```python
from build123d import *

# Parameters (mm, degrees)
SKETCH3_R           = 0.405
BOSS_EXTRUDE2_DEPTH = 70


with BuildPart() as part:
    # Sketch2 → Revolve1 (revolve)
    with BuildSketch(Plane.XY):
        Polygon((0, 0), (-9.85, 0), (-9.85, 4.95), (-3.328991597, 4.95), (-3.328991597, 5.45), (0, 5.45), align=None)
    revolve(axis=Axis((0, 5.45, 0), (0, -1, 0)))

    # Sketch3 → Boss-Extrude2 (add)
    with BuildSketch(Plane(origin=(0, 0, 0), x_dir=(0, 0, -1), z_dir=(1, 0, 0))):
        with Locations(Location((-0.41, 2.05, 0), (0, 0, 180))):
            Circle(SKETCH3_R)
        with Locations(Location((-1.23, 2.05, 0), (0, 0, 180))):
            Circle(SKETCH3_R)
        with Locations(Location((1.23, 2.05, 0), (0, 0, 180))):
            Circle(SKETCH3_R)
        with Locations(Location((0.41, 2.05, 0), (0, 0, 180))):
            Circle(SKETCH3_R)
    extrude(amount=BOSS_EXTRUDE2_DEPTH)


solid = part.part
```
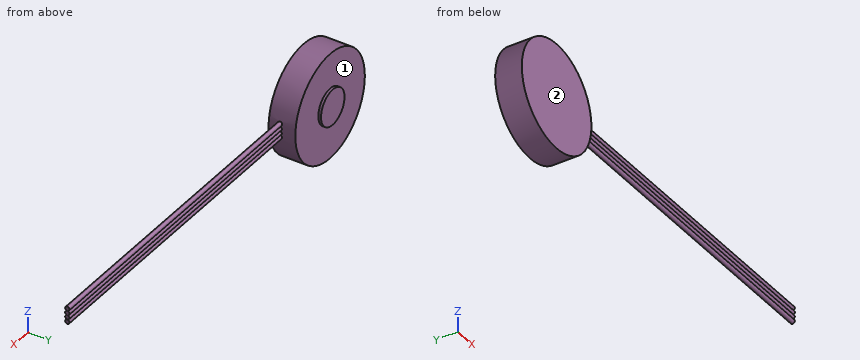
CAD build for the part. Positions are in the model's coordinates, mm. Face numbers are marked on the shaded views. A direction names the side the tool comes from. Give positions to 0.01 mm unless a question says otherwise; leave off trailing zeros. Write each loop counter-clockwise with the first axis right and the second up, starting at its lowest first coordinate (ties: lowest second). Pieces come first, ordered by that corner, then holes. Notation, with made-up numbers: M 5.25,39.5 L 9.25,39.5 A27 cw 9.25,59.5 Z; hole C -12.5,-26.75 d2. An arc over 180 degrees is marked long. Return JSON: item names as keys, results as strings. Group by question number.
(1) Flat gauge pins, fed straight in: pin 1 Ø3 at (x, y) = (26, 2) entering from +Z (3 decimals); pin 2 Ø10 at (x, z) = (16.5, -6) entering from +Y (3 decimals); pin 3 Ø1 at (x, z) = (20, -4) entering from -Y; pin 4 Ø1.5 at (x, y) = (-1.5, 4) entering from -Z. Where does each tip first touch, or does it go through?
(2) Drill centre lines: L1, parallel to Z at x = 34.5, y = 1.75; L2, parallel to Z at x = 33, y = 1.8; L3, parallel to Z at x = 0.5, y = 4.6. Where is each one in solid material? Low to high. Write a range as [from, to].
(3) Band-saw the part on C-C (y = 4.2). Give the cut face in (x, z), and give its area (3 significant figures).
(4) Band-saw the part on D-D (z = 4.75). Give the cut face in (x, y), and give its area (3 significant figures).
(5) Band-saw the part on B-B (x = 62.5). Give the cut face in (y, z) (3 decimals).
(6) Band-saw the part on A-A (x = 0). Give the cut face in (y, z).
(7) 3-axis set-ups, long thin cutter, end or side, ignore diameter. For the marked faces 1 and 2: which of +Z, -Z, +X, -X, +Y, -Y reach the whole face in a straight line?
Entries:
{
 "1": {"pin 1": "stops at z = 1.635", "pin 2": "stops at y = 2.455", "pin 3": "passes through", "pin 4": "stops at z = -9.82"},
 "2": {"L1": "z = [-1.5, -0.96], [-0.68, -0.14], [0.14, 0.68], [0.96, 1.5]", "L2": "z = [-1.55, -0.91], [-0.73, -0.09], [0.09, 0.73], [0.91, 1.55]", "L3": "z = [-9.84, 9.84]"},
 "3": {"outline": "C 0,0 d19.7", "area": "305 mm^2"},
 "4": {"outline": "M -8.63,0 L 8.63,0 L 8.63,4.95 L -8.63,4.95 Z", "area": "85.4 mm^2"},
 "5": {"outline": "C 2.05,-1.23 d0.81; C 2.05,-0.41 d0.81; C 2.05,0.41 d0.81; C 2.05,1.23 d0.81"},
 "6": {"outline": "M 0,-9.85 L 4.95,-9.85 L 4.95,-3.33 L 5.45,-3.33 L 5.45,3.33 L 4.95,3.33 L 4.95,9.85 L 0,9.85 Z"},
 "7": {"face 1": "+Y", "face 2": "+Z, -Z, +X, -X, -Y"}
}
